Read the model definition and answer for the solid it produces. Units are mm, in the model's axes. A direction names the side the tool comes from. Give positions to 0.01 mm unless a question says otherwise; leave off trailing zeros. Write each loop counter-clockwise with the first axis right and the second up, starting at its lowest first coordinate (ties: lowest second). Pieces come first, ordered by that corner, then holes. Notation, with made-up numbers: M 40.25,-17 L 57.25,-17 A35 cw 57.25,22 Z; hole C -38.5,5.25 d1. An arc over 180 degrees is marked long. Put each result on its own line as item: value.
from build123d import *

# Parameters (mm, degrees)
F0_R     = 3.25
F1_DEPTH = 15
F2_R     = 1.75
F3_DEPTH = 9
F5_R     = 1.75
F6_DEPTH = 4


with BuildPart() as f1:
    # F0 (on Top) → F1 (new body)
    with BuildSketch(Plane.XY):
        Circle(F0_R)
    extrude(amount=F1_DEPTH)

    # F2 (on face) → F3 (cut)
    with BuildSketch(Plane(origin=(0, 0, 0), x_dir=(1, 0, 0), z_dir=(0, 0, -1))):
        Circle(F2_R)
    extrude(amount=-F3_DEPTH, mode=Mode.SUBTRACT)

    # F5 (on offset) → F6 (cut)
    with BuildSketch(Plane(origin=(0, 0, 10), x_dir=(1, 0, 0), z_dir=(0, 0, -1))):
        Circle(F5_R)
    extrude(amount=-F6_DEPTH, mode=Mode.SUBTRACT)


solid = f1.part
(1) Section C-C on z = 9.75 is taken. Determine the outline of the cut face in (x, y).
Result:
outline: C 0,0 d6.5
(2) Section B-B on x = -1 is taken. Determine the outline of the cut face in (y, z).
Result:
outline: M -3.09,0 L -1.44,0 L -1.44,9 L 1.44,9 L 1.44,0 L 3.09,0 L 3.09,15 L -3.09,15 Z; hole M -1.44,10 L 1.44,10 L 1.44,14 L -1.44,14 Z
(3) Straight lines are drawn through the part: line 1 along Y through (x, z) = (0, 6); line 2 along Z through (x, y) = (0, 0); line 3 along X through (y, z) = (1, 10.75). For each, find the intervals that lie inside material, in ascending order. Write a range as from..to.
Result:
line 1: y = -3.25..-1.75, 1.75..3.25
line 2: z = 9..10, 14..15
line 3: x = -3.09..-1.44, 1.44..3.09
(4) Section A-A on y = 0 is taken. Determine the outline of the cut face in (x, z), and give its area (3 significant figures).
Result:
outline: M -3.25,0 L -1.75,0 L -1.75,9 L 1.75,9 L 1.75,0 L 3.25,0 L 3.25,15 L -3.25,15 Z; hole M -1.75,10 L 1.75,10 L 1.75,14 L -1.75,14 Z
area: 52.0 mm²
(5) Which of the six approach directions +Z, -Z, +X, -X, +Y, -Y give full straight-line access (tool end or side, diameter ignored) to faces 4 (the face through (1.617, 0.67, 4.437)), 5 (the face through (0, 0, 15)), 6 (the face through (0, 0, 14))?
Result:
face 4: -Z
face 5: +Z, +X, -X, +Y, -Y
face 6: none
(6) Section D-D on y = -3 is taken. Determine the outline of the cut face in (x, z).
Result:
outline: M -1.25,0 L 1.25,0 L 1.25,15 L -1.25,15 Z
(7) For a pull along Z with two mould halves and no side action, classify faces 1 (the face through (1.4, -1.4, 0)), 2 (the face through (-2.579, -1.978, 7.395)), 3 (the face through (1.617, 0.67, 11.972)) as +Z half, -Z half, draft (parallel to the pull), parting line (faces both ways), or undercut.
Result:
face 1: -Z half
face 2: draft
face 3: undercut
(8) Given pin 1 Ø2 at (x, y) = (0, 0) entering from -Z; pin 2 Ø2 at (y, z) = (2.5, 7.5) entering from +X; pin 3 Ø3 at (y, z) = (2, 4) entering from +X; pin 4 Ø1.8 at (x, y) = (0.5, -1) entering from -Z, each flat-ended and moving along its own axis, determine where each tip first touches the part or whether it passes through.
Result:
pin 1: stops at z = 9
pin 2: stops at x = 2.88
pin 3: stops at x = 3.21
pin 4: stops at z = 0
